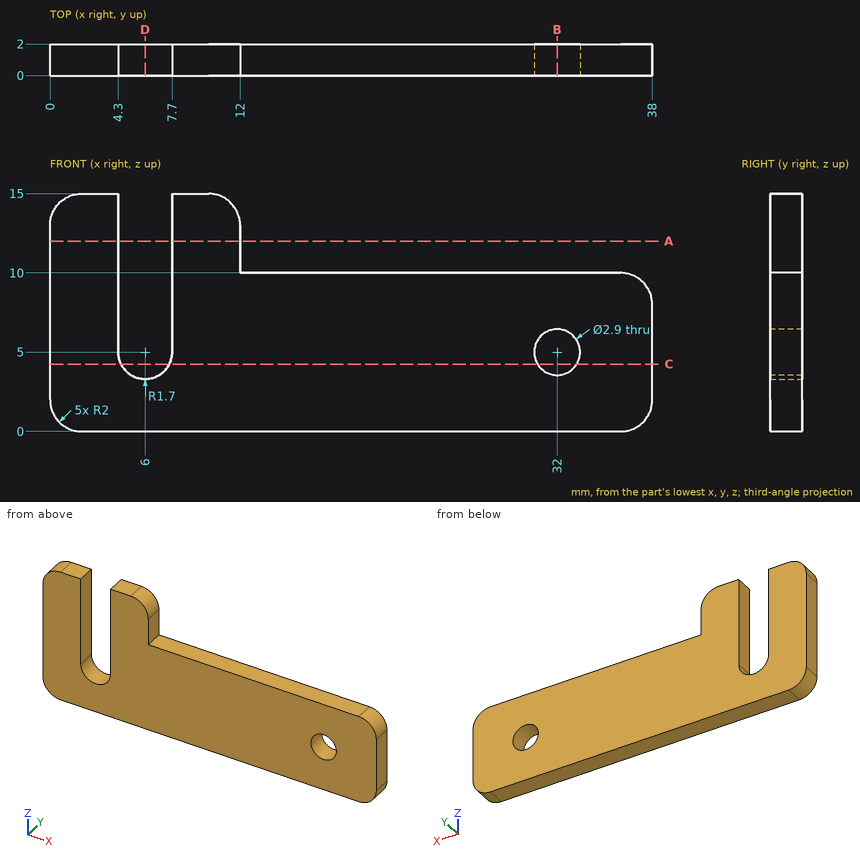
The figure shows three views and two pictorial views of one solid part (mm, origin at its lowest corner). Answer the questions. Give positions to 0.01 mm unless a question says otherwise; leave off trailing zeros. Order: outer loops, then holes, each group sorted by start corner. A loop starts at its lowest first (then second) coordinate and runs counter-clockwise, first axis right, second up. Notation, with made-up numbers: (-37.75, -5) -> (14.25, -5) arc R20 cw to (14.25, 8) -> close; hole circle Ø5 at (-23, 60.5). An arc over 180 degrees is marked (long way). Answer as CSV lines item,"result". Start each with the question number.
Q1. A cutting plane is placed at D-D (x = 6). Determine the outline of the cut face in (y, z), then the cut area to 3 significant figures.
Q2. Find the intervals of material crossed by L1, parallel to X at y = 0.55, z = 5; L2, parallel to Z at x = 32, y = 0.75; L3, parallel to X at y = 0.15, z = 11, in increasing order.
Q3. Given pin 1 (3.5 mm diameter, centred on x = 32, z = 5, fed in from -Y); pin 2 (0.6 mm diameter, centred on y = 1.5, z = 12, fed in from +X), each flat-ended and moving along its own axis, determine where each tip first touches the part or whether it passes through.
Q4. A cutting plane is placed at C-C (z = 4.25). Determine the outline of the cut face in (x, y), then the cut area to 3 significant figures.
Q5. A cutting plane is placed at B-B (x = 32). Determine the outline of the cut face in (y, z), then the cut area to 3 significant figures.
Q6. A cutting plane is placed at A-A (z = 12). Determine the outline of the cut face in (x, y).
Results found:
1,outline,"(0, 0) -> (2, 0) -> (2, 3.3) -> (0, 3.3) -> close"
1,area,"6.60 mm2"
2,L1,"0 to 4.3, 7.7 to 30.55, 33.45 to 38"
2,L2,"0 to 3.55, 6.45 to 10"
2,L3,"0 to 4.3, 7.7 to 12"
3,pin 1,"y = 0"
3,pin 2,"x = 12"
4,outline,"(0, 0) -> (4.47, 0) -> (4.47, 2) -> (0, 2) -> close; (7.53, 0) -> (30.76, 0) -> (30.76, 2) -> (7.53, 2) -> close; (33.24, 0) -> (38, 0) -> (38, 2) -> (33.24, 2) -> close"
4,area,"64.9 mm2"
5,outline,"(0, 0) -> (2, 0) -> (2, 3.55) -> (0, 3.55) -> close; (0, 6.45) -> (2, 6.45) -> (2, 10) -> (0, 10) -> close"
5,area,"14.2 mm2"
6,outline,"(0, 0) -> (4.3, 0) -> (4.3, 2) -> (0, 2) -> close; (7.7, 0) -> (12, 0) -> (12, 2) -> (7.7, 2) -> close"
